Can you work these out from the drawing? Everything is in mm from the part's minimum corner. Round coordinates to 2 decimals unless told otherwise and drop trailing zeros. Order: outer loops, then holes, each group sorted by start corner. A loop starts at its lowest first (then second) coordinate and runs counter-clockwise, first axis right, second up. Notation, with made-up numbers: (-15.75, 88) -> (22.25, 88) arc R24 ccw to (22.25, 105) -> close; hole circle Ø3 at (43, 73.25). An arc over 180 degrees is marked (long way). One line per item, written item: value.
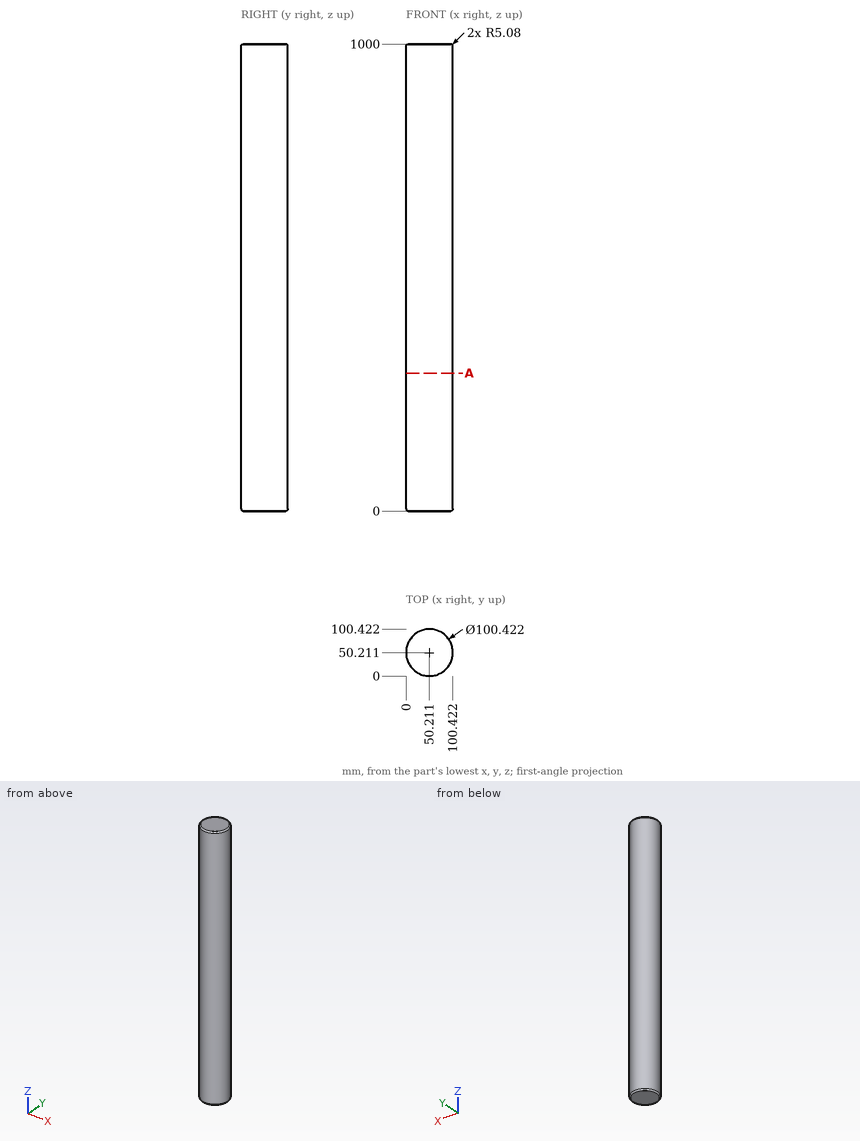
Q1. Will these pins go through, and if not, where does the flat tip stop? pin 1 Ø1.5 at (x, z) = (57.5, 301) entering from +Y (1 decimal); pin 2 Ø1 at (y, z) = (14, 784) entering from -X (1 decimal); pin 3 Ø8 at (y, z) = (11, 177) entering from +X.
Answers below:
pin 1: y = 100
pin 2: x = 14.9
pin 3: x = 86.01
Q2. Please list where these lines run through material, in increasing order: line 1 along Y through (x, z) = (53.5, 298) (1 decimal); line 2 along Y through (x, z) = (49.5, 390) (1 decimal); line 3 along X through (y, z) = (52, 90).
Answers below:
line 1: 0.1 to 100.3
line 2: 0 to 100.4
line 3: 0.03 to 100.39
Q3. I want a section at A-A on z = 295.5. List the corners of the cut face in (x, y) for me, plus the area to 3 significant figures.
Answers below:
outline: circle Ø100.42 at (50.21, 50.21)
area: 7,920 mm^2
